Build history of the part. All positions in model axes, mm. Round coordinates to 2 decimals unless told otherwise and drop trailing zeros. Write each loop counter-clockwise with the first axis right and the second up, starting at its lowest first coordinate (ties: lowest second). Pieces come first, ordered by that corner, then holes.
from build123d import *

# Parameters (mm, degrees)
CYLINDER408_R     = 5
CYLINDER408_DEPTH = 100
CYLINDER409_R     = 5
CYLINDER409_DEPTH = 100
CYLINDER410_R     = 5
CYLINDER410_DEPTH = 100
CYLINDER411_R     = 5
CYLINDER411_DEPTH = 100
CYLINDER412_R     = 5
CYLINDER412_DEPTH = 100
CYLINDER413_R     = 5
CYLINDER413_DEPTH = 100
CYLINDER414_R     = 5
CYLINDER414_DEPTH = 100
CYLINDER407_R     = 5
CYLINDER407_DEPTH = 100
BOX134_W          = 10
BOX134_H          = 108
BOX134_DEPTH      = 50
CHAMFER_SIZE      = 5


with BuildPart() as obj1:
    # Cylinder408 → Cylinder408 (new body)
    with BuildSketch(Plane(origin=(24, -51, 25), x_dir=(0, 0, -1), z_dir=(1, 0, 0))):
        Circle(CYLINDER408_R)
    extrude(amount=CYLINDER408_DEPTH)


with BuildPart() as obj2:
    # Cylinder409 → Cylinder409 (new body)
    with BuildSketch(Plane(origin=(24, 36, 34), x_dir=(0, 0, -1), z_dir=(1, 0, 0))):
        Circle(CYLINDER409_R)
    extrude(amount=CYLINDER409_DEPTH)


with BuildPart() as obj3:
    # Cylinder410 → Cylinder410 (new body)
    with BuildSketch(Plane(origin=(24, -36, 34), x_dir=(0, 0, -1), z_dir=(1, 0, 0))):
        Circle(CYLINDER410_R)
    extrude(amount=CYLINDER410_DEPTH)


with BuildPart() as obj4:
    # Cylinder411 → Cylinder411 (new body)
    with BuildSketch(Plane(origin=(24, -23, -5), x_dir=(0, 0, -1), z_dir=(1, 0, 0))):
        Circle(CYLINDER411_R)
    extrude(amount=CYLINDER411_DEPTH)


with BuildPart() as obj5:
    # Cylinder412 → Cylinder412 (new body)
    with BuildSketch(Plane(origin=(24, 51, 7), x_dir=(0, 0, -1), z_dir=(1, 0, 0))):
        Circle(CYLINDER412_R)
    extrude(amount=CYLINDER412_DEPTH)


with BuildPart() as obj6:
    # Cylinder413 → Cylinder413 (new body)
    with BuildSketch(Plane(origin=(24, 23, -5), x_dir=(0, 0, -1), z_dir=(1, 0, 0))):
        Circle(CYLINDER413_R)
    extrude(amount=CYLINDER413_DEPTH)


with BuildPart() as obj7:
    # Cylinder414 → Cylinder414 (new body)
    with BuildSketch(Plane(origin=(24, -51, 7), x_dir=(0, 0, -1), z_dir=(1, 0, 0))):
        Circle(CYLINDER414_R)
    extrude(amount=CYLINDER414_DEPTH)


with BuildPart() as compound586:
    # Cylinder407 → Cylinder407 (new body)
    with BuildSketch(Plane(origin=(24, 51, 25), x_dir=(0, 0, -1), z_dir=(1, 0, 0))):
        Circle(CYLINDER407_R)
    extrude(amount=CYLINDER407_DEPTH)

    # Compound586: union obj1, obj2, obj3, obj4, obj5, obj6, obj7
    add(obj1.part)
    add(obj2.part)
    add(obj3.part)
    add(obj4.part)
    add(obj5.part)
    add(obj6.part)
    add(obj7.part)


with BuildPart() as compound586_1:
    # Compound586 placement: moved
    add(compound586.part.moved(Location((32, 0, 0))))


with BuildPart() as cut362:
    # Box134 → Box134 (new body)
    with BuildSketch(Plane(origin=(87, -29, -8), x_dir=(1, 0, 0), z_dir=(0, 0, 1))):
        with Locations((5, 54)):
            Rectangle(BOX134_W, BOX134_H)
    extrude(amount=BOX134_DEPTH)

    # Chamfer
    chamfer_edges = [cut362.edges().sort_by_distance(p)[0] for p in [
        (87, 25, 42),
    ]]
    chamfer(chamfer_edges, length=CHAMFER_SIZE)

    # Cut362: cut Compound586
    add(compound586_1.part, mode=Mode.SUBTRACT)


solid = cut362.part
1) Slice it at D-D (z = 7). Write the cut outline in (x, y), plus the area to 3 significant figures.
Results:
outline: (87, -29) - (97, -29) - (97, 46) - (87, 46) - close; (87, 56) - (97, 56) - (97, 79) - (87, 79) - close
area: 980 mm2
2) Slice it at C-C (y = 51). Write the cut outline in (x, z).
Results:
outline: (87, -8) - (97, -8) - (97, 2) - (87, 2) - close; (87, 12) - (97, 12) - (97, 20) - (87, 20) - close; (87, 30) - (97, 30) - (97, 42) - (92, 42) - (87, 37) - close
3) Slice it at A-A (x = 94). Write the cut outline in (y, z).
Results:
outline: (-29, -8) - (-27, -8) arc R5 cw (long way) to (-19, -8) - (19, -8) arc R5 cw (long way) to (27, -8) - (79, -8) - (79, 42) - (-29, 42) - close; hole circle Ø10 at (36, 34); hole circle Ø10 at (51, 7); hole circle Ø10 at (51, 25)
4) Wall check: L1, parallel to Y at x = 93.5, z = -5; L2, parallel to Z at x = 93.5, y = 51; L3, parallel to Z at x = 89.5, y = 51. Give the ranges that are in metal, low to high.
Results:
L1: y = -29 to -28, -18 to 18, 28 to 79
L2: z = -8 to 2, 12 to 20, 30 to 42
L3: z = -8 to 2, 12 to 20, 30 to 39.5
5) Slice it at B-B (y = 33). Write the cut outline in (x, z).
Results:
outline: (87, -8) - (97, -8) - (97, 30) - (87, 30) - close; (88, 38) - (97, 38) - (97, 42) - (92, 42) - close
6) Mould opens along Y. For faces 1 (the cylindrical face through (92, 23, 0)), 2 (the cylindrical face through (92, 55, 4)), 3 (the flat face through (92, -29, 17)), 4 (the flat face through (92, -28, -8)) say: released by +Y, released by -Y, zero draft, split by the parting line, or undercut.
Results:
face 1: undercut
face 2: undercut
face 3: released by -Y
face 4: zero draft
